Check sheet for the drawn part. Datum: minimum x, y, z corner. Units: mm. Give positions to 0.01 mm unless a question says otherwise; leave off trailing zeros. Order: outer loops, then holes, each group sorted by start corner. A loop starts at its lowest first (then second) coordinate and runs counter-clockwise, first axis right, second up. Notation, with made-up numbers: M 47.25,1 L 51.25,1 A5 cw 51.25,6 Z; hole C 89,-39 d1. An arc over 180 degrees is marked long. Answer as CSV lines item,"result". Start each with the question number.
Q1. Go/stop test with flat-tipped pins: pin 1 (2 mm diameter, centred on x = 395, z = 11.5, fed in from +Y); pin 2 (1.5 mm diameter, centred on x = 173, z = 14.5, fed in from -Y); pin 3 (8 mm diameter, centred on x = 396, y = 397, fed in from +Z); pin 4 (10 mm diameter, centred on x = 454, y = 239.5, fed in from +Z). Record where each tip stops, or that it passes through.
Q2. Section check C-C, the plane y = 454. Record the boundary of the cut face in (x, z), then the cut area to 3 significant figures.
Q3. Section check A-A, the plane y = 239.5. Record the boundary of the cut face in (x, z), then the cut area to 3 significant figures.
Q4. Thickness scan on line 1 (Y direction, x = 239, z = 25); line 2 (X direction, y = 389, z = 13) (1 decimal); line 3 (Y direction, x = 118, z = 10). Record the ranges inside material, lowest first.
Q5. Section check B-B, the plane x = 268.5. Record the boundary of the cut face in (y, z), then the cut area to 3 significant figures.
Q6. Mould release check, pull along X, two halves, no side actions. Record for the marked faces 1, 2 and 3: +X half, -X half, draft (parallel to the pull), parting line (faces both ways), or undercut.
Q7. Section check D-D, the plane x = 320. Record the boundary of the cut face in (y, z), then the cut area to 3 significant figures.
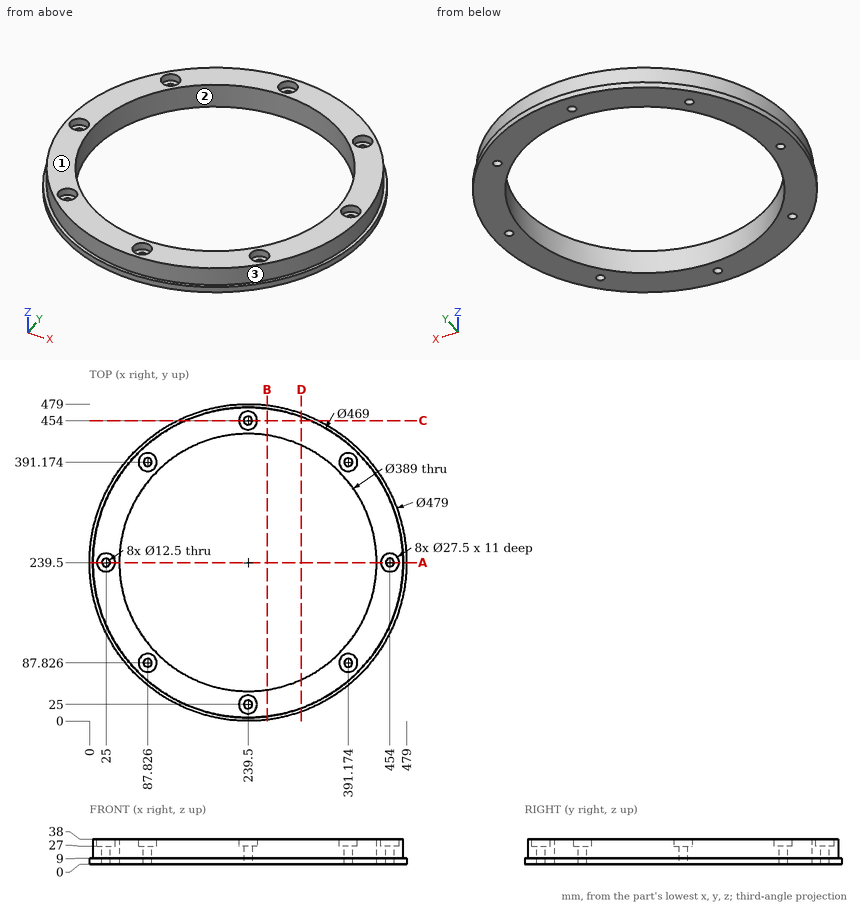
Answer block:
1,pin 1,"stops at y = 415.91"
1,pin 2,"stops at y = 14.41"
1,pin 3,"stops at z = 27"
1,pin 4,"passes through"
2,outline,"M 132.96,0 L 233.25,0 L 233.25,27 L 225.75,27 L 225.75,38 L 144.74,38 L 144.74,9 L 132.96,9 Z; M 245.75,0 L 346.04,0 L 346.04,9 L 334.26,9 L 334.26,38 L 253.25,38 L 253.25,27 L 245.75,27 Z"
2,area,"6,770 mm2"
3,outline,"M 0,0 L 18.75,0 L 18.75,27 L 11.25,27 L 11.25,38 L 5,38 L 5,9 L 0,9 Z; M 31.25,0 L 45,0 L 45,38 L 38.75,38 L 38.75,27 L 31.25,27 Z; M 434,0 L 447.75,0 L 447.75,27 L 440.25,27 L 440.25,38 L 434,38 Z; M 460.25,0 L 479,0 L 479,9 L 474,9 L 474,38 L 467.75,38 L 467.75,27 L 460.25,27 Z"
3,area,"1,850 mm2"
4,line 1,"y = 5 to 18.77, 31.23 to 45, 434 to 447.77, 460.23 to 474"
4,line 2,"x = 58.8 to 82, 93.7 to 115.1, 363.9 to 385.3, 397 to 420.2"
4,line 3,"y = 38.93 to 87.62, 391.38 to 440.07"
5,outline,"M 1.76,0 L 47.17,0 L 47.17,38 L 6.8,38 L 6.8,9 L 1.76,9 Z; M 431.83,0 L 477.24,0 L 477.24,9 L 472.2,9 L 472.2,38 L 431.83,38 Z"
5,area,"3,160 mm2"
6,face 1,"draft"
6,face 2,"undercut"
6,face 3,"parting line"
7,outline,"M 13.93,0 L 62.44,0 L 62.44,38 L 19.25,38 L 19.25,9 L 13.93,9 Z; M 416.56,0 L 465.07,0 L 465.07,9 L 459.75,9 L 459.75,38 L 416.56,38 Z"
7,area,"3,380 mm2"
